from build123d import *

# Parameters (mm, degrees)
SKETCH1_R               = 142.875
SKETCH1_R_2             = 11.25
BOSS_EXTRUDE2_DEPTH     = 3.81
SKETCH2_R               = 9.779
CUT_EXTRUDE1_DEPTH      = 203.091680556
CUT_EXTRUDE2_DEPTH      = 203.091680556
CUT_EXTRUDE2_DEPTH_BACK = 203.091680556
FILLET1_R               = 12.7
CIRPATTERN1_COUNT       = 32
SKETCH5_R               = 2.5
CUT_EXTRUDE3_DEPTH      = 203.091680556


with BuildPart() as part:
    # Sketch1 → Boss-Extrude2 (new body)
    with BuildSketch(Plane(origin=(0, 0, 0), x_dir=(1, 0, 0), z_dir=(0, 1, 0))):
        with Locations(Location((0, 0, 0), (0, 0, 270))):
            Circle(SKETCH1_R)
        with Locations(Location((0, 0, 0), (0, 0, 270))):
            Circle(SKETCH1_R_2, mode=Mode.SUBTRACT)
    extrude(amount=-BOSS_EXTRUDE2_DEPTH)

    # Sketch2 → Cut-Extrude1 (cut, through all)
    with BuildSketch(Plane(origin=(0, 0, 0), x_dir=(1, 0, 0), z_dir=(0, 1, 0))):
        with Locations(Location((-127, 0, 0), (0, 0, 270))):
            Circle(SKETCH2_R)
    cut_extrude1 = extrude(amount=-CUT_EXTRUDE1_DEPTH, mode=Mode.SUBTRACT)

    # Sketch4 → Cut-Extrude2 (cut, two sides: drawn at the far end of the back side and taken through both)
    with BuildSketch(Plane(origin=(0, 0, 0), x_dir=(1, 0, 0), z_dir=(0, 1, 0)).offset(-CUT_EXTRUDE2_DEPTH_BACK)):
        with BuildLine():
            ThreePointArc((10.795, -110.59942857), (78.577241059, -78.577241059), (110.59942857, -10.795))
            Line((110.59942857, -10.795), (14.330567107, -10.795))
            Line((14.330567107, -10.795), (10.795, -10.795))
            Line((10.795, -10.795), (10.795, -14.276272178))
            Line((10.795, -14.276272178), (10.795, -110.59942857))
        make_face()
        with BuildLine():
            ThreePointArc((110.59942857, 10.795), (78.577241059, 78.577241059), (10.795, 110.59942857))
            Line((10.795, 110.59942857), (10.795, 13.38498083))
            Line((10.795, 13.38498083), (10.795, 10.795))
            Line((10.795, 10.795), (14.557306927, 10.795))
            Line((14.557306927, 10.795), (110.59942857, 10.795))
        make_face()
        with BuildLine():
            Line((-10.795, 10.795), (-10.795, 16.346811669))
            Line((-10.795, 16.346811669), (-10.795, 110.59942857))
            ThreePointArc((-10.795, 110.59942857), (-78.577241059, 78.577241059), (-110.59942857, 10.795))
            Line((-110.59942857, 10.795), (-13.320463431, 10.795))
            Line((-13.320463431, 10.795), (-10.795, 10.795))
        make_face()
        with BuildLine():
            Line((-15.550882255, -10.795), (-110.59942857, -10.795))
            ThreePointArc((-110.59942857, -10.795), (-78.577241059, -78.577241059), (-10.795, -110.59942857))
            Line((-10.795, -110.59942857), (-10.795, -14.068746807))
            Line((-10.795, -14.068746807), (-10.795, -10.795))
            Line((-10.795, -10.795), (-15.550882255, -10.795))
        make_face()
    extrude(amount=CUT_EXTRUDE2_DEPTH + CUT_EXTRUDE2_DEPTH_BACK, mode=Mode.SUBTRACT)

    # Fillet1
    fillet1_edges = [part.edges().sort_by_distance(p)[0] for p in [
        (-110.59942857, -1.905, 10.795),
        (-10.795, -1.905, 10.795),
        (-10.795, -1.905, 110.59942857),
        (-10.795, -1.905, -110.59942857),
        (-10.795, -1.905, -10.795),
        (-110.59942857, -1.905, -10.795),
        (110.59942857, -1.905, -10.795),
        (10.795, -1.905, -10.795),
        (10.795, -1.905, -110.59942857),
        (10.795, -1.905, 110.59942857),
        (10.795, -1.905, 10.795),
        (110.59942857, -1.905, 10.795),
    ]]
    fillet(fillet1_edges, radius=FILLET1_R)

    # CirPattern1: Cut-Extrude1 ×32 about axis
    cirpattern1_axis = Axis((0, 0, 0), (0, 1, 0))
    for i in range(1, CIRPATTERN1_COUNT):
        add(cut_extrude1.rotate(cirpattern1_axis, i * 360 / CIRPATTERN1_COUNT), mode=Mode.SUBTRACT)

    # Sketch5 → Cut-Extrude3 (cut, through all)
    with BuildSketch(Plane(origin=(0, 0, 0), x_dir=(1, 0, 0), z_dir=(0, 1, 0))):
        with Locations(Location((0, 47.5, 0), (0, 0, 270))):
            Circle(SKETCH5_R)
        with Locations(Location((47.5, 0, 0), (0, 0, 270))):
            Circle(SKETCH5_R)
        with Locations(Location((0, -47.5, 0), (0, 0, 270))):
            Circle(SKETCH5_R)
        with Locations(Location((-47.5, 0, 0), (0, 0, 270))):
            Circle(SKETCH5_R)
    extrude(amount=-CUT_EXTRUDE3_DEPTH, mode=Mode.SUBTRACT)


solid = part.part
CAD build for the part. Positions are in the model's coordinates, mm. Coordinates: 2 decimals unless noted, no trailing zeros. Write each loop counter-clockwise with the first axis right and the second up, starting at its lowest first coordinate (ties: lowest second). Pieces come first, ordered by that corner, then holes. Notation, with made-up numbers: (-40, 11) - (-34, 11) arc R26 cw to (-34, 32) - close; hole circle Ø2 at (39, 87.25). An arc over 180 degrees is marked (long way). Use a Markdown table: item, result. Add a question column.
Item 1: Mould opens along Z. For faces 1 (the face through (42.916, -1.878, 136.277)), 2 (the face through (-101.661, -1.878, -61.605)) say: pulls with the +Z half, pulls with the -Z half, needs draft (parallel to the pull), parting line crosses it, or undercut.
Item 2: Band-saw the part on A-A, the plane x = 104. Give the cut face in (y, z).
Item 3: Drill centre lines: L1, parallel to X at y = -1.8, z = 94.5 (3 decimals); L2, parallel to Z at x = 54.5, y = -0.9 (3 decimals); L3, parallel to X at y = -3.05, z = -4. Where is each one in solid material? Low to high. Write a range as from..to.
Item 4: Band-saw the part on C-C, the plane y = -0.7. Give the number of separate pieces and of enclosed holes in the cut face, and give its area (3 significant figures).
Item 5: Band-saw the part on B-B, the plane z = 92. Give the cut face in (x, y) (3 decimals).
Item 6: Flat gauge pins, fed straight in: pin 1 (8 mm diameter, centred on x = -93.5, z = 86, fed in from -Y); pin 2 (1.1 mm diameter, centred on y = -2, z = 58, fed in from -X); pin 3 (1 mm diameter, centred on y = -2, z = -27, fed in from +X); pin 4 (1.5 mm diameter, centred on x = -59.5, y = -0.5, fed in from +Z). Where does each tip first touch, or does it go through?
Numbers:
| question | item | result |
|---|---|---|
| 1 | face 1 | parting line crosses it |
| 1 | face 2 | undercut |
| 2 | outline | (-3.81, -97.97) - (0, -97.97) - (0, -80.21) - (-3.81, -80.21) - close; (-3.81, -60.91) - (0, -60.91) - (0, -39.15) - (-3.81, -39.15) - close; (-3.81, -13.99) - (0, -13.99) - (0, 13.99) - (-3.81, 13.99) - close; (-3.81, 39.15) - (0, 39.15) - (0, 60.91) - (-3.81, 60.91) - close; (-3.81, 80.21) - (0, 80.21) - (0, 97.97) - (-3.81, 97.97) - close |
| 3 | L1 | -107.159..-98.379, -81.226..-58.468, -10.795..10.795, 58.468..81.226, 98.379..107.159 |
| 3 | L2 | -132.072..-125.132, -109.533..-96.843, -10.795..10.795, 96.843..109.533, 125.132..132.072 |
| 3 | L3 | -142.82..-135.92, -118.08..-10.51, 10.51..118.08, 135.92..142.82 |
| 4 | separate pieces | 1 |
| 4 | enclosed holes | 41 |
| 4 | area | 24,900 mm2 |
| 5 | outline | (-109.313, -3.81) - (-99.331, -3.81) - (-99.331, 0) - (-109.313, 0) - close; (-80.274, -3.81) - (-62.328, -3.81) - (-62.328, 0) - (-80.274, 0) - close; (-10.795, -3.81) - (10.795, -3.81) - (10.795, 0) - (-10.795, 0) - close; (62.328, -3.81) - (80.274, -3.81) - (80.274, 0) - (62.328, 0) - close; (99.331, -3.81) - (109.313, -3.81) - (109.313, 0) - (99.331, 0) - close |
| 6 | pin 1 | through |
| 6 | pin 2 | x = -130.82 |
| 6 | pin 3 | x = 140.4 |
| 6 | pin 4 | z = 130.24 |
